Verification items for the finished model (mm, model axes). Face numbers are marked on the shaded views. A direction names the side the tool comes from. Round coordinates to 2 decimals unless told otherwise and drop trailing zeros. Order: outer loops, then holes, each group sorted by start corner. A loop starts at its lowest first (then second) coordinate and runs counter-clockwise, first axis right, second up. Notation, with made-up numbers: (74, 17.25) -> (78, 17.25) arc R31 cw to (78, 55.25) -> close; hole circle Ø4 at (42.25, -10.75). An arc over 180 degrees is marked (long way). Answer in a Markdown table with one row per item. Add a question column.
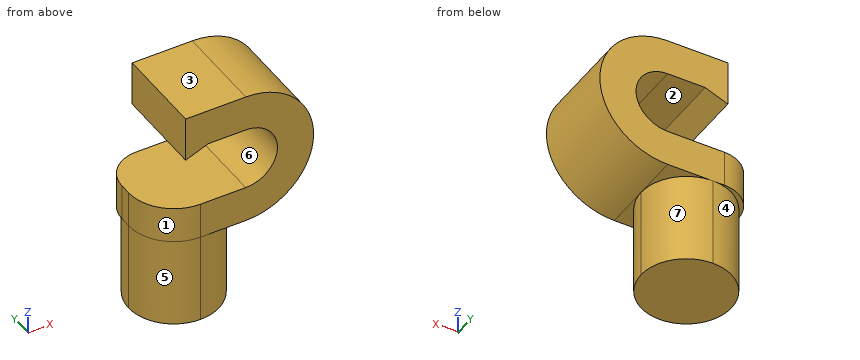
Autodesk Inventor part; units mm, degrees
ref_plane "YZ Plane" through (0, 0, 0) normal (1, 0, 0) x (0, 1, 0)
ref_plane "XZ Plane" through (0, 0, 0) normal (0, 1, 0) x (-1, 0, 0)
ref_plane "XY Plane" through (0, 0, 0) normal (0, 0, 1) x (1, 0, 0)
sketch "Sketch1" plane through (0, 0, 0) normal (0, 0, 1) x (1, 0, 0)
  line L0 (0, 0) -> (12.7, 0)
  line L1 (12.7, 0) -> (12.7, -12.7)
  line L2 (12.7, -12.7) -> (0, -12.7)
  line L3 (0, -12.7) -> (0, 0)
  point P0 (6.35, -12.7)
  point P1 (6.35, 0)
  dimension "d0" = 12.7
  dimension "d1" = 12.7
extrude "Extrusion1" add sketch "Sketch1" along normal blind 12.7
fillet "Fillet1" radius 6.35 4 edges at (12.7, 0, 6.35) (0, 0, 6.35) (0, -12.7, 6.35) (12.7, -12.7, 6.35)
sketch "Sketch2" plane through (6.35, -6.35, 12.7) normal (0, 0, 1) x (1, 0, 0)
  line L0 (-2.0483, -0.0105) -> (1.7617, -0.0105)
  line L1 (1.7617, -0.0105) -> (1.7617, -0.03)
  line L2 (1.7617, -0.03) -> (-2.0483, -0.03)
  line L3 (-2.0483, -0.03) -> (-2.0483, -0.0105)
  point P0 (-6.35, 6.35)
extrude "Extrusion2" add sketch "Sketch2" along normal blind 2.54
sketch "Sketch4" plane through (4.3017, -6.3605, 12.7) normal (0, 1, 0) x (1, 0, 0)
  line L0 (8.3983, 0) -> (-4.3017, 0)
  arc A0 (8.3983, -19.05) -> (8.3983, 0) centre (8.3983, -9.525) ccw
  line L1 (8.3983, -19.05) -> (-0.04, -19.05)
  line L2 (-0.04, -19.05) -> (-0.04, -13.97)
  line L3 (-0.04, -13.97) -> (8.3983, -13.97)
  line L4 (-4.3017, 0) -> (-4.3017, -5.08)
  line L5 (-4.3017, -5.08) -> (8.3983, -5.08)
  arc A1 (8.3983, -13.97) -> (8.3983, -5.08) centre (8.3983, -9.525) ccw
  point P0 (-4.3017, 12.7)
  dimension "d10" = 19.05
  dimension "d11" = 5.08
  dimension "d12" = 5.08
extrude "Extrusion3" add sketch "Sketch4" along normal mid plane 12.7
fillet "Fillet2" radius 6.35 1 edges at (0, -12.7105, 15.24)
fillet "Fillet3" radius 4.7625 1 edges at (0, -0.0105, 15.24)
sketch "Sketch5" plane through (12.7, -0.0105, 26.67) normal (0, 0, -1) x (-1, 0, 0)
  line L0 (0, 0) -> (8.4383, 0)
  line L1 (8.4383, -12.7) -> (0, -12.7)
  line L2 (8.4383, 0) -> (5.2633, 0)
  line L3 (5.2633, 0) -> (5.2633, -12.7)
  line L4 (5.2633, -12.7) -> (8.4383, -12.7)
  line L5 (8.4383, -12.7) -> (8.4383, 0)
  point P0 (12.7, 0.0105)
  point P1 (5.2633, 0)
  dimension "d17" = 3.175
extrude "Extrusion4" add sketch "Sketch5" along normal blind 1.27
chamfer "Chamfer1" distance 3.175 angle 21.8 1 edges at (7.4367, -6.3605, 25.4) measured on face at (6.3784, -4.2438, 25.4)
properties part number "Hitch to the Polar Express [Copy]"
1) Thickness scan on L1, parallel to Z at x = 11.25, y = -10; L2, parallel to Z at x = 12.5, y = -1; L3, parallel to Y at x = 16.5, z = 18.5. Record the ranges inside material, lowest first. Write a range as [from, to].
2) Cross-section at B-B, the plane x = 10.5. Record the boundary of the cut face in (y, z).
3) Depth check by flat-ended pin: P1, Ø2, axis at x = 4, z = 6.5, coming from the +Y side; P2, Ø12, axis at x = 17.5, z = 10, coming from the +Y side; P3, Ø1.5, axis at y = -9, z = 26.5, coming from the +X side; P4, Ø4, axis at x = 16, z = 6, coming from the -Y side. Enter the tip coordinate at first touch or a pass-through.
4) Tool access check on the marked faces 4, 5, 6 and 7. Record the directions out of +Z, -Z, +X, -X, +Y, -Y that give a thin tool (end or side, any length) a straight path to the whole face; none if there is none.
5) Draft check along Z on the marked faces 1, 2 and 3. Enter one of: +Z half, -Z half, draft (parallel to the pull), parting line (faces both ways), or undercut.
Results below:
| question | item | result |
|---|---|---|
| 1 | L1 | [0, 17.78], [26.67, 31.75] |
| 1 | L2 | [12.7, 17.78], [26.67, 31.75] |
| 1 | L3 | [-12.71, -0.01] |
| 2 | outline | (-12.71, 12.7) -> (-11.16, 12.7) -> (-11.16, 0) -> (-1.54, 0) -> (-1.54, 12.7) -> (-0.01, 12.7) -> (-0.01, 17.78) -> (-12.71, 17.78) -> close; (-12.71, 26.67) -> (-0.01, 26.67) -> (-0.01, 31.75) -> (-12.71, 31.75) -> close |
| 3 | P1 | y = -0.15 |
| 3 | P2 | y = -0.01 |
| 3 | P3 | x = 21.55 |
| 3 | P4 | through |
| 4 | face 4 | -Z, -X, +Y |
| 4 | face 5 | -Z, -X, -Y |
| 4 | face 6 | +Y, -Y |
| 4 | face 7 | -Z, +X, +Y |
| 5 | face 1 | draft |
| 5 | face 2 | undercut |
| 5 | face 3 | +Z half |
